Autodesk Inventor part; units mm, degrees
ref_plane "YZ Plane" through (0, 0, 0) normal (1, 0, 0) x (0, 1, 0)
ref_plane "XZ Plane" through (0, 0, 0) normal (0, 1, 0) x (-1, 0, 0)
ref_plane "XY Plane" through (0, 0, 0) normal (0, 0, 1) x (1, 0, 0)
sketch "Esquisse1" plane through (0, 0, 0) normal (0, 0, 1) x (1, 0, 0)
  line L0 (0, 0) -> (18.3, 0)
  line L1 (18.3, 0) -> (18.3, 2.2)
  line L2 (18.3, 2.2) -> (-2.2, 2.2)
  line L3 (-2.2, 2.2) -> (-2.2, -18.3)
  line L4 (-2.2, -18.3) -> (0, -18.3)
  line L5 (0, -18.3) -> (0, 0)
  dimension "Epaisseur_cornière" = 2.2
  dimension "Largueur" = 20.5
extrude "Embase" add sketch "Esquisse1" along normal mid plane 310.4
sketch "Esquisse2" plane through (0, 0, 0) normal (0, 1, 0) x (-1, 0, 0)
  line L0 (2.2, 155.2) -> (-18.3, 134.7)
  line L1 (-18.3, 134.7) -> (-18.3, 155.2)
  line L2 (-18.3, 155.2) -> (2.2, 155.2)
  line L3 (-18.3, 155.2) -> (2.2, 155.2) construction
  line L4 (2.2, -155.2) -> (2.2, 155.2) construction
  line L5 (-18.3, -155.2) -> (-18.3, 155.2) construction
  point P0 (0, 0)
  dimension "d4" = 45
extrude "Découpe à 45" cut sketch "Esquisse2" along normal through all both and the other way through all
mirror "Symétrie découpe" about plane through (0, 0, 0) normal (0, 0, 1) of "Découpe à 45"
properties part number "Profilé superieur cote" material "Aluminium 6061"
For this review, take the finished solid that the model builds, in its own axes (mm). A direction names the side the tool comes from. Round coordinates to 2 decimals unless told otherwise and drop trailing zeros. Write each loop counter-clockwise with the first axis right and the second up, starting at its lowest first coordinate (ties: lowest second). Pieces come first, ordered by that corner, then holes. Notation, with made-up numbers: M 57.25,77 L 72.25,77 A4 ccw 72.25,83 Z; hole C 52,56 d11. An arc over 180 degrees is marked long. One line per item, written item: value. Start each with the question number.
(1) Insertion check: pin 1 (5 mm diameter, centred on y = -14.5, z = -117, fed in from +X); pin 2 (1 mm diameter, centred on x = 0, y = 0, fed in from -Z). Each pin has a flat end and moves straight along its axis. Give the tip position at first contact, or say it passes through.
(2) We need section A-A (z = -6.5). Give the boundary of the cut face in (x, y).
(3) Wall thickness on line 1 (X direction, y = -2.5, z = 17); line 2 (Y direction, x = 5.75, z = -49): over which ranges is each line inside the solid? List them lowest first.
(4) Machinability: for faces 1 (the flat face through (3.5, 0.3, -149.5)), 2 (the flat face through (9, 0, -2)), which of the approach directions +Z, -Z, +X, -X, +Y, -Y give a long, thin tool a straight path to every point of the face, cutting with its end or side? Answer none if there is none.
(5) We need section C-C (x = 11.75). Give the boundary of the cut face in (y, z).
(6) We need section B-B (y = -13.5). Give the boundary of the cut face in (x, z), and give its area (3 significant figures).
Result:
1. pin 1: x = 0
1. pin 2: z = -153.5
2. outline: M -2.2,-18.3 L 0,-18.3 L 0,0 L 18.3,0 L 18.3,2.2 L -2.2,2.2 Z
3. line 1: -2.2 to 0
3. line 2: 0 to 2.2
4. face 1: -Z, +X, +Y, -Y
4. face 2: +Z, -Z, +X, -Y
5. outline: M 0,-141.25 L 2.2,-141.25 L 2.2,141.25 L 0,141.25 Z
6. outline: M -2.2,-155.2 L 0,-153 L 0,153 L -2.2,155.2 Z
6. area: 678 mm²
